Part model, mm, in its own coordinate system. Round coordinates to 2 decimals unless told otherwise and drop trailing zeros. Loops run counter-clockwise (first coordinate to the right, second up) from the corner with the lowest first, then second, coordinate; pieces in that order, holes last.
1) Probe line 1 (X direction, y = -11.5, z = 17.75); line 2 (Z direction, x = -41.5, y = -14); line 3 (Y direction, x = -24.5, z = 9.5). List the from-to ranges inside material, lowest first.
2) Band-saw the part on A-A, the plane x = -38.75. Write the cut outline in (y, z), then the cut area to 3 significant figures.
3) Band-saw the part on B-B, the plane z = 9. Write the cut outline in (x, y).
from build123d import *

# Parameters (mm, degrees)
F0_W     = 18.796
F0_H     = 18.796
F1_DEPTH = 18.796
F2_SIZE2 = 2
F2_SIZE  = 2


with BuildPart() as f1:
    # F0 (on Top) → F1 (new body)
    with BuildSketch(Plane.XY):
        with Locations((-33.203556, -17.694149)):
            Rectangle(F0_W, F0_H)
    extrude(amount=F1_DEPTH)

    # F2
    f2_edges = [f1.edges().sort_by_distance(p)[0] for p in [
        (-42.601556, -17.694149, 18.796),
        (-33.203556, -27.092149, 18.796),
        (-42.601556, -27.092149, 9.398),
        (-42.601556, -8.296149, 9.398),
        (-42.601556, -17.694149, 0),
        (-33.203556, -27.092149, 0),
        (-23.805556, -27.092149, 9.398),
        (-33.203556, -8.296149, 18.796),
        (-23.805556, -8.296149, 9.398),
        (-23.805556, -17.694149, 0),
        (-23.805556, -17.694149, 18.796),
        (-33.203556, -8.296149, 0),
    ]]
    chamfer(f2_edges, length=F2_SIZE, length2=F2_SIZE2)


solid = f1.part
Reported:
1. line 1: x = -41.65 to -24.76
1. line 2: z = 0.9 to 17.9
1. line 3: y = -25.79 to -9.6
2. outline: (-27.09, 2) - (-25.09, 0) - (-10.3, 0) - (-8.3, 2) - (-8.3, 16.8) - (-10.3, 18.8) - (-25.09, 18.8) - (-27.09, 16.8) - close
2. area: 345 mm2
3. outline: (-42.6, -25.09) - (-40.6, -27.09) - (-25.81, -27.09) - (-23.81, -25.09) - (-23.81, -10.3) - (-25.81, -8.3) - (-40.6, -8.3) - (-42.6, -10.3) - close
